```python
from build123d import *

# Parameters (mm, degrees)
BOSS_EXTRU_1_DEPTH = 53.5
CONG_1_R           = 3


with BuildPart() as part:
    # Esquisse1 → Boss.-Extru.1 (new body, symmetric)
    with BuildSketch(Plane.XY):
        with BuildLine():
            Line((-11.3, 0), (11.3, 0))
            Line((11.3, 0), (11.3, -40))
            Line((11.3, -40), (15.3, -40))
            ThreePointArc((15.3, -40), (25.272141163, 7.430887623), (53.5, 46.830388705))
            Line((53.5, 46.830388705), (-53.5, 46.830388705))
            ThreePointArc((-53.5, 46.830388705), (-25.272141163, 7.430887623), (-15.3, -40))
            Line((-15.3, -40), (-11.3, -40))
            Line((-11.3, -40), (-11.3, 0))
        make_face()
        with BuildLine():
            Line((43.806234565, 42.830388705), (-43.806234565, 42.830388705))
            ThreePointArc((-43.806234565, 42.830388705), (-26.353615228, 18.651434723), (-15.3, -9.043931817))
            Line((-15.3, -9.043931817), (-15.3, 4))
            Line((-15.3, 4), (15.3, 4))
            Line((15.3, 4), (15.3, -9.043931817))
            ThreePointArc((15.3, -9.043931817), (26.353615228, 18.651434723), (43.806234565, 42.830388705))
        make_face(mode=Mode.SUBTRACT)
    extrude(amount=BOSS_EXTRU_1_DEPTH, both=True)

    # Congé1
    cong_1_edges = [part.edges().sort_by_distance(p)[0] for p in [
        (0, 46.830388705, 53.5),
        (-15.3, -40, 0),
        (-53.5, 46.830388705, 0),
        (53.5, 46.830388705, 0),
        (15.3, -40, 0),
        (0, 46.830388705, -53.5),
        (0, 4, -53.5),
        (15.3, 4, 0),
        (-15.3, 4, 0),
        (0, 4, 53.5),
    ]]
    fillet(cong_1_edges, radius=CONG_1_R)


solid = part.part
```
Build history of the part. All positions in model axes, mm. A direction names the side the tool comes from. Round coordinates to 2 decimals unless told otherwise and drop trailing zeros. Write each loop counter-clockwise with the first axis right and the second up, starting at its lowest first coordinate (ties: lowest second). Pieces come first, ordered by that corner, then holes. Notation, with made-up numbers: (21.5, -13.75) - (75.5, -13.75) arc R15 cw to (75.5, 3.25) - close; hole circle Ø11 at (0, 8). An arc over 180 degrees is marked (long way). Answer as CSV lines item,"result".
Q1. Cut at A-A (z = -45). Write the cut outline in (x, y).
Report:
outline,"(-48.29, 41.75) arc R117.78 cw to (-15.34, -37.07) arc R3 ccw to (-12.34, -40) - (-11.3, -40) - (-11.3, 0) - (11.3, 0) - (11.3, -40) - (12.34, -40) arc R3 ccw to (15.34, -37.07) arc R117.78 cw to (48.29, 41.75) arc R3 ccw to (46.13, 46.83) - (-46.13, 46.83) arc R3 ccw to start; hole (-43.81, 42.83) arc R121.78 cw to (-15.3, -9.04) - (-15.3, 1) arc R3 cw to (-12.3, 4) - (12.3, 4) arc R3 cw to (15.3, 1) - (15.3, -9.04) arc R121.78 cw to (43.81, 42.83) - close"
Q2. Cut at B-B (x = 1). Write the cut outline in (y, z).
Report:
outline,"(0, -53.5) - (1, -53.5) arc R3 ccw to (4, -50.5) - (4, 50.5) arc R3 ccw to (1, 53.5) - (0, 53.5) - close; (42.83, -53.5) - (43.83, -53.5) arc R3 ccw to (46.83, -50.5) - (46.83, 50.5) arc R3 ccw to (43.83, 53.5) - (42.83, 53.5) - close"
Q3. Pull direction X, two halves, no side cores. Call faces 6 (the cylindrical face through (-48.908, 44.958, -0.749)), 7 (the cylindrical face through (48.87, 45.05, 0.75)), 8 (the flat face through (15.3, -4, 1)): +X half, -X half, draft (parallel to the pull), parting line (faces both ways), or undercut.
Report:
face 6,"-X half"
face 7,"+X half"
face 8,"undercut"
Q4. Drill centre lines: probe 1 along Y at (x, z) = (0, -25.5); probe 2 along X at (y, z) = (-5.5, -12); probe 3 along Y at (x, z) = (-29.5, 5.5). Where is each one in solid material? Low to high. Write a range as [from, to].
Report:
probe 1,"y = [0, 4], [42.83, 46.83]"
probe 2,"x = [-20.47, -16.29], [-15.3, -11.3], [11.3, 15.3], [16.29, 20.47]"
probe 3,"y = [16.07, 24.04], [42.83, 46.83]"
Q5. Cut at C-C (y = 20). Write the cut outline in (x, z).
Report:
outline,"(-31.73, -53.5) - (-27.11, -53.5) - (-27.11, 53.5) - (-31.73, 53.5) - close; (27.11, -53.5) - (31.73, -53.5) - (31.73, 53.5) - (27.11, 53.5) - close"
Q6. Tool access for faces 1 (the flat face through (1, 42.83, 1)), 2 (the cylindrical face through (-14.41, -39.17, -0.75)), 3 (the flat face through (1, 46.83, 1)), 4 (the flat face through (11.3, -20, 1)), 5 (the cylindrical face through (0.21, 3.1, 52.64)): list every direction of +Z, -Z, +X, -X, +Y, -Y with a clear straight run to the whole face (end or side of a thin tool).
Report:
face 1,"+Z, -Z"
face 2,"+Z, -Z, -X, -Y"
face 3,"+Z, -Z, +X, -X, +Y"
face 4,"+Z, -Z, -Y"
face 5,"+Z"
Q7. Cut at D-D (y = -24.5). Write the cut outline in (x, z), and give its area (3 significant figures).
Report:
outline,"(-16.32, -53.5) - (-11.3, -53.5) - (-11.3, 53.5) - (-16.32, 53.5) - close; (11.3, -53.5) - (16.32, -53.5) - (16.32, 53.5) - (11.3, 53.5) - close"
area,"1,080 mm^2"
Q8. Drop flat-ended pins along their axis: pin 1 (11.5 mm diameter, centred on x = 4.5, z = 5.5, fed in from -Y); pin 2 (6 mm diameter, centred on y = 5.5, z = -28.5, fed in from -X); pin 3 (1 mm diameter, centred on y = 34.5, z = -7, fed in from +X). Give the stop position or say it passes through.
Report:
pin 1,"stops at y = 0"
pin 2,"stops at x = -25.75"
pin 3,"stops at x = 42.26"
